from build123d import *

# Parameters (mm, degrees)
BOSS_EXTRUDE1_DEPTH                    = 38.1
BOSS_EXTRUDE1_DEPTH_BACK               = 2
SKETCH1_W                              = 165.1
SKETCH1_H                              = 165.1
SKETCH2_W                              = 95.25
SKETCH2_H                              = 95.25
BOSS_EXTRUDE2_DEPTH                    = 38.1
BOSS_EXTRUDE5_DEPTH                    = 95.1
SKETCH5_R                              = 12.7
CUT_EXTRUDE1_DEPTH                     = 198.290297523
SKETCH6_W                              = 38.1
SKETCH6_H                              = 85.0398732
CUT_EXTRUDE2_DEPTH                     = 198.290297523
FILLET1_R                              = 3.175
SKETCH7_R                              = 26
CUT_EXTRUDE3_DEPTH                     = 36.83
SKETCH8_R                              = 76.2
SKETCH8_R_2                            = 69.85
CUT_EXTRUDE4_DEPTH                     = 8
F_1_2_14_NPSM_TAPPED_HOLE1_D           = 18.9738
F_1_2_14_NPSM_TAPPED_HOLE1_DEPTH       = 63.5
F_1_2_14_NPSM_TAPPED_HOLE1_CSINK_D     = 22.1742
F_1_2_14_NPSM_TAPPED_HOLE1_CSINK_ANGLE = 90
F_1_2_14_NPSM_TAPPED_HOLE1_TIP         = 5.700304607
SKETCH15_R                             = 6.35
BOSS_EXTRUDE6_DEPTH                    = 30
SKETCH16_R                             = 6.35
CUT_EXTRUDE5_DEPTH                     = 25
SKETCH17_R                             = 6.35
CUT_EXTRUDE6_DEPTH                     = 172.14027248


with BuildPart() as part:
    # Sketch1 → Boss-Extrude1 (new, two sides: drawn at the far end of the back side and taken through both)
    with BuildSketch(Plane(origin=(0, 0, 0), x_dir=(1, 0, 0), z_dir=(0, 1, 0)).offset(-BOSS_EXTRUDE1_DEPTH_BACK)):
        Rectangle(SKETCH1_W, SKETCH1_H)
    extrude(amount=BOSS_EXTRUDE1_DEPTH + BOSS_EXTRUDE1_DEPTH_BACK)

    # Sketch2 → Boss-Extrude2 (add)
    with BuildSketch(Plane(origin=(0, 38.1, 0), x_dir=(1, 0, 0), z_dir=(0, 1, 0))):
        Rectangle(SKETCH2_W, SKETCH2_H)
    extrude(amount=BOSS_EXTRUDE2_DEPTH)

    # Sketch4 → Boss-Extrude5 (add)
    with BuildSketch(Plane.XY.offset(47.625)):
        with BuildLine():
            Line((-47.625, 76.2), (47.625, 76.2))
            ThreePointArc((47.625, 76.2), (0, 123.1398732), (-47.625, 76.2))
        make_face()
    extrude(amount=-BOSS_EXTRUDE5_DEPTH)

    # Sketch5 → Cut-Extrude1 (cut, through all)
    with BuildSketch(Plane.XY.offset(47.625)):
        with Locations((0, 76.643842778)):
            Circle(SKETCH5_R)
    extrude(amount=-CUT_EXTRUDE1_DEPTH, mode=Mode.SUBTRACT)

    # Sketch6 → Cut-Extrude2 (cut, through all)
    with BuildSketch(Plane.ZY.offset(47.625)):
        with Locations((-0.1412698, 80.6199366)):
            Rectangle(SKETCH6_W, SKETCH6_H)
    extrude(amount=-CUT_EXTRUDE2_DEPTH, mode=Mode.SUBTRACT)

    # Fillet1
    fillet1_edges = [part.edges().sort_by_distance(p)[0] for p in [
        (82.55, 18.05, 82.55),
        (-82.55, 18.05, 82.55),
        (-82.55, 18.05, -82.55),
        (82.55, 18.05, -82.55),
    ]]
    fillet(fillet1_edges, radius=FILLET1_R)

    # Sketch7 → Cut-Extrude3 (cut)
    with BuildSketch(Plane.XZ.offset(2)):
        with Locations(Location((0, 0, 0), (0, 0, 270))):
            Circle(SKETCH7_R)
    extrude(amount=-CUT_EXTRUDE3_DEPTH, mode=Mode.SUBTRACT)

    # Sketch8 → Cut-Extrude4 (cut)
    with BuildSketch(Plane.XZ.offset(2)):
        with Locations(Location((0, 0, 0), (0, 0, 270))):
            Circle(SKETCH8_R)
        with Locations(Location((0, 0, 0), (0, 0, 270))):
            Circle(SKETCH8_R_2, mode=Mode.SUBTRACT)
    extrude(amount=-CUT_EXTRUDE4_DEPTH, mode=Mode.SUBTRACT)

    # 1/2-14 NPSM Tapped Hole1
    with Locations(Plane(origin=(82.55, 0, 0), x_dir=(0, 0, -1), z_dir=(1, 0, 0))):
        with Locations((0, 18.05)):
            CounterSinkHole(F_1_2_14_NPSM_TAPPED_HOLE1_D / 2, F_1_2_14_NPSM_TAPPED_HOLE1_CSINK_D / 2, depth=F_1_2_14_NPSM_TAPPED_HOLE1_DEPTH, counter_sink_angle=F_1_2_14_NPSM_TAPPED_HOLE1_CSINK_ANGLE)
            with Locations((0, 0, -(F_1_2_14_NPSM_TAPPED_HOLE1_DEPTH + F_1_2_14_NPSM_TAPPED_HOLE1_TIP / 2))):  # 118° drill point
                Cone(0, F_1_2_14_NPSM_TAPPED_HOLE1_D / 2, F_1_2_14_NPSM_TAPPED_HOLE1_TIP, mode=Mode.SUBTRACT)

    # Sketch15 → Boss-Extrude6 (add)
    with BuildSketch(Plane.XZ.offset(2)):
        with Locations(Location((50.301871098, 0, 0), (0, 0, 270))):
            Circle(SKETCH15_R)
    extrude(amount=-BOSS_EXTRUDE6_DEPTH)

    # Sketch16 → Cut-Extrude5 (cut)
    with BuildSketch(Plane.XZ.offset(2)):
        with Locations(Location((50.55, 0, 0), (0, 0, 270))):
            Circle(SKETCH16_R)
    extrude(amount=-CUT_EXTRUDE5_DEPTH, mode=Mode.SUBTRACT)

    # Sketch17 → Cut-Extrude6 (cut, through all)
    with BuildSketch(Plane.XZ.offset(2)):
        with Locations(Location((-68.538631425, 54.602865331, 0), (0, 0, 270))):
            Circle(SKETCH17_R)
        with Locations(Location((68.538631425, 54.602865331, 0), (0, 0, 270))):
            Circle(SKETCH17_R)
        with Locations(Location((-68.538631425, -54.602865331, 0), (0, 0, 270))):
            Circle(SKETCH17_R)
        with Locations(Location((68.538631425, -54.602865331, 0), (0, 0, 270))):
            Circle(SKETCH17_R)
    extrude(amount=-CUT_EXTRUDE6_DEPTH, mode=Mode.SUBTRACT)


solid = part.part
Work out the finished part from the listing and answer in its coordinate system (mm). A direction names the side the tool comes from. Coordinates: 2 decimals unless noted, no trailing zeros. Loops run counter-clockwise (first coordinate to the right, second up) from the corner with the lowest first, then second, coordinate; pieces in that order, holes last. Notation, with made-up numbers: (20, 25) -> (31, 25) arc R28 ccw to (31, 47) -> close; hole circle Ø9 at (48, -4). An arc over 180 degrees is marked (long way). Write each question's results on one line, items separated by ' | '. Start each with the question number.
1) For faces 5 (the cylindrical face through (-68.2, 1.9, 15.1)), 6 (the flat face through (-0.7, 89.5, -19.191)), 7 (the flat face through (-1, 91, 47.625)), determine the directions among +Z, -Z, +X, -X, +Y, -Y from which every point of the face is accessible in a straight line to the end or side of a thin tool.
2) Find section C-C on y = 45.5. Determine the outline of the cut face in (x, z) (3 decimals).
3) Consider line 1 along Z through (x, y) = (13, 84) (3 decimals); line 2 along Y through (x, z) = (0, -41); line 3 along Y through (x, z) = (33, -10). Determine where each line is inside the solid, lowest interval first.
4) Flat-ended cylindrical pins translate along their axes: P1, Ø14.5, axis at x = -68.54, z = -54.6, coming from the +Y side; P2, Ø2, axis at x = 22.5, y = 99.5, coming from the -Z side (3 decimals); P3, Ø1, axis at x = -2.5, y = 57, coming from the +Z side (3 decimals). Find the tip coordinate at first contact, or state that the pin passes through.
5) The mould has two halves that part along X. Classify faces 1 (the cylindrical face through (-1.653, 89.236, -33.209)), 2 (the cylindrical face through (-46.367, 1.944, 60.47)), 3 (the flat face through (-82.55, 18, 1)), 4 (the cylindrical face through (1.04, 123.13, 33.47)): pulls with the +X half, pulls with the -X half, needs draft (parallel to the pull), parting line crosses it, or undercut.
6) Find section D-D on y = 18.05. Determine the outline of the cut face in (x, z) (3 decimals), then the cut area to 3 significant figures.
7) Find section A-A on x = 0. Count the separate pieces of the cut face and the enclosed holes in it, then the cut area to 3 significant figures.
Response values:
1) face 5: -Y | face 6: +X, -X, +Y | face 7: +Z, +X, -X, +Y
2) outline: (-47.625, -47.625) -> (47.625, -47.625) -> (47.625, -19.191) -> (-47.625, -19.191) -> close; (-47.625, 18.909) -> (47.625, 18.909) -> (47.625, 47.625) -> (-47.625, 47.625) -> close
3) line 1: z = -47.475 to -19.191, 18.909 to 47.625 | line 2: y = -2 to 63.94, 89.34 to 123.14 | line 3: y = -2 to 38.1
4) P1: stops at y = 38.1 | P2: stops at z = -47.475 | P3: stops at z = 47.625
5) face 1: undercut | face 2: undercut | face 3: pulls with the -X half | face 4: parting line crosses it
6) outline: (-82.55, -79.375) arc R3.175 ccw to (-79.375, -82.55) -> (79.375, -82.55) arc R3.175 ccw to (82.55, -79.375) -> (82.55, -11.087) -> (80.95, -9.487) -> (24.207, -9.487) arc R26 cw (long way) to (24.207, 9.487) -> (80.95, 9.487) -> (82.55, 11.087) -> (82.55, 79.375) arc R3.175 ccw to (79.375, 82.55) -> (-79.375, 82.55) arc R3.175 ccw to (-82.55, 79.375) -> close; (50.426, -6.349) arc R6.35 cw to (50.426, 6.349) arc R6.35 ccw (long way) to start; hole circle Ø12.7 at (-68.539, -54.603); hole circle Ø12.7 at (-68.539, 54.603); hole circle Ø12.7 at (68.539, -54.603); hole circle Ø12.7 at (68.539, 54.603) | area: 23,500 mm^2
7) separate pieces: 3 | enclosed holes: 0 | area: 8,010 mm^2
